from build123d import *

# Parameters (mm, degrees)
SKETCH_1_W          = 20
SKETCH_1_H          = 20
SKETCH_1_W_2        = 17
SKETCH_1_H_2        = 17
EXTRUDE_1_DEPTH     = 250
SKETCH_2_R          = 2.1
SKETCH_2_R_2        = 1.6
CUT_EXTRUDE_1_DEPTH = 251.99800796
SKETCH_3_R          = 4
CUT_EXTRUDE_3_DEPTH = 251.99800796


with BuildPart() as part:
    # 草图1 → 凸台-拉伸1 (new body)
    with BuildSketch(Plane.XY):
        Rectangle(SKETCH_1_W, SKETCH_1_H)
        Rectangle(SKETCH_1_W_2, SKETCH_1_H_2, mode=Mode.SUBTRACT)
    extrude(amount=EXTRUDE_1_DEPTH)

    # 草图2 → 切除-拉伸1 (cut, through all)
    with BuildSketch(Plane(origin=(0, 10, 0), x_dir=(1, 0, 0), z_dir=(0, 1, 0))):
        with Locations(Location((0, -7.5, 0), (0, 0, 270))):
            Circle(SKETCH_2_R)
        with Locations(Location((0, -22.5, 0), (0, 0, 270))):
            Circle(SKETCH_2_R)
        with Locations(Location((0, -120, 0), (0, 0, 270))):
            Circle(SKETCH_2_R_2)
        with Locations((0, -130)):
            Circle(SKETCH_2_R_2)
        with Locations((0, -227.5)):
            Circle(SKETCH_2_R)
        with Locations((0, -242.5)):
            Circle(SKETCH_2_R)
    extrude(amount=-CUT_EXTRUDE_1_DEPTH, mode=Mode.SUBTRACT)

    # 草图3 → 切除-拉伸3 (cut, through all)
    with BuildSketch(Plane.ZY.offset(10)):
        with Locations((197, 0)):
            Circle(SKETCH_3_R)
        with Locations(Location((53, 0, 0), (0, 0, 270))):
            Circle(SKETCH_3_R)
    extrude(amount=-CUT_EXTRUDE_3_DEPTH, mode=Mode.SUBTRACT)


solid = part.part
Verification items for the finished model (mm, model axes). A direction names the side the tool comes from. Coordinates: 2 decimals unless noted, no trailing zeros. Loops run counter-clockwise (first coordinate to the right, second up) from the corner with the lowest first, then second, coordinate; pieces in that order, holes last. Notation, with made-up numbers: (54.5, -31) -> (85.5, -31) arc R29 cw to (85.5, 8) -> close; hole circle Ø6 at (54.5, 24.5). An arc over 180 degrees is marked (long way). Write each question's results on one line, items separated by ' | '.
Item 1: Gauge pin test, flat end, axial feed: pin 1 (1.5 mm diameter, centred on x = -6, y = 6, fed in from +Z). Record the tip position at first contact, or that the pin passes through.
Found:
pin 1: passes through
Item 2: Section check B-B, the plane x = -6. Enter the section's corners in (y, z), plus the area to 3 significant figures.
Found:
outline: (-10, 0) -> (-8.5, 0) -> (-8.5, 250) -> (-10, 250) -> close; (8.5, 0) -> (10, 0) -> (10, 250) -> (8.5, 250) -> close | area: 750 mm2
Item 3: Section check C-C, the plane z = 37. Enter the section's corners in (x, y), plus the area to 3 significant figures.
Found:
outline: (-10, -10) -> (10, -10) -> (10, 10) -> (-10, 10) -> close; hole (-8.5, -8.5) -> (8.5, -8.5) -> (8.5, 8.5) -> (-8.5, 8.5) -> close | area: 111 mm2
Item 4: Section check A-A, the plane z = 197. Enter the section's corners in (x, y), plus the area to 3 significant figures.
Found:
outline: (-10, -10) -> (10, -10) -> (10, -4) -> (8.5, -4) -> (8.5, -8.5) -> (-8.5, -8.5) -> (-8.5, -4) -> (-10, -4) -> close; (-10, 4) -> (-8.5, 4) -> (-8.5, 8.5) -> (8.5, 8.5) -> (8.5, 4) -> (10, 4) -> (10, 10) -> (-10, 10) -> close | area: 87.0 mm2
Item 5: Section check D-D, the plane z = 227.5. Enter the section's corners in (x, y).
Found:
outline: (-10, -10) -> (-2.1, -10) -> (-2.1, -8.5) -> (-8.5, -8.5) -> (-8.5, 8.5) -> (-2.1, 8.5) -> (-2.1, 10) -> (-10, 10) -> close; (2.1, -10) -> (10, -10) -> (10, 10) -> (2.1, 10) -> (2.1, 8.5) -> (8.5, 8.5) -> (8.5, -8.5) -> (2.1, -8.5) -> close
Item 6: Material ranges on L1, parallel to X at y = 9, z = 242.5; L2, parallel to X at y = 6.5, z = 126.5, recorded low to high.
Found:
L1: x = -10 to -2.1, 2.1 to 10 | L2: x = -10 to -8.5, 8.5 to 10
Item 7: Tool access check on faces 5 (the face through (0.09, -9.24, 5.4)), 6 (the face through (0, -8.5, 123)). Record the directions out of +Z, -Z, +X, -X, +Y, -Y that give a thin tool (end or side, any length) a straight path to the whole face; none if there is none.
Found:
face 5: +Y, -Y | face 6: +Z, -Z
Item 8: Mould release check, pull along Z, two halves, no side actions. Record for faces 1 (the face through (-9, 0, 250)), 2 (the face through (0.09, 9.26, 5.4)), 3 (the face through (-8.5, 0, 123)), 4 (the face through (-9, 0, 0)): +Z half, -Z half, draft (parallel to the pull), parting line (faces both ways), or undercut.
Found:
face 1: +Z half | face 2: undercut | face 3: draft | face 4: -Z half
